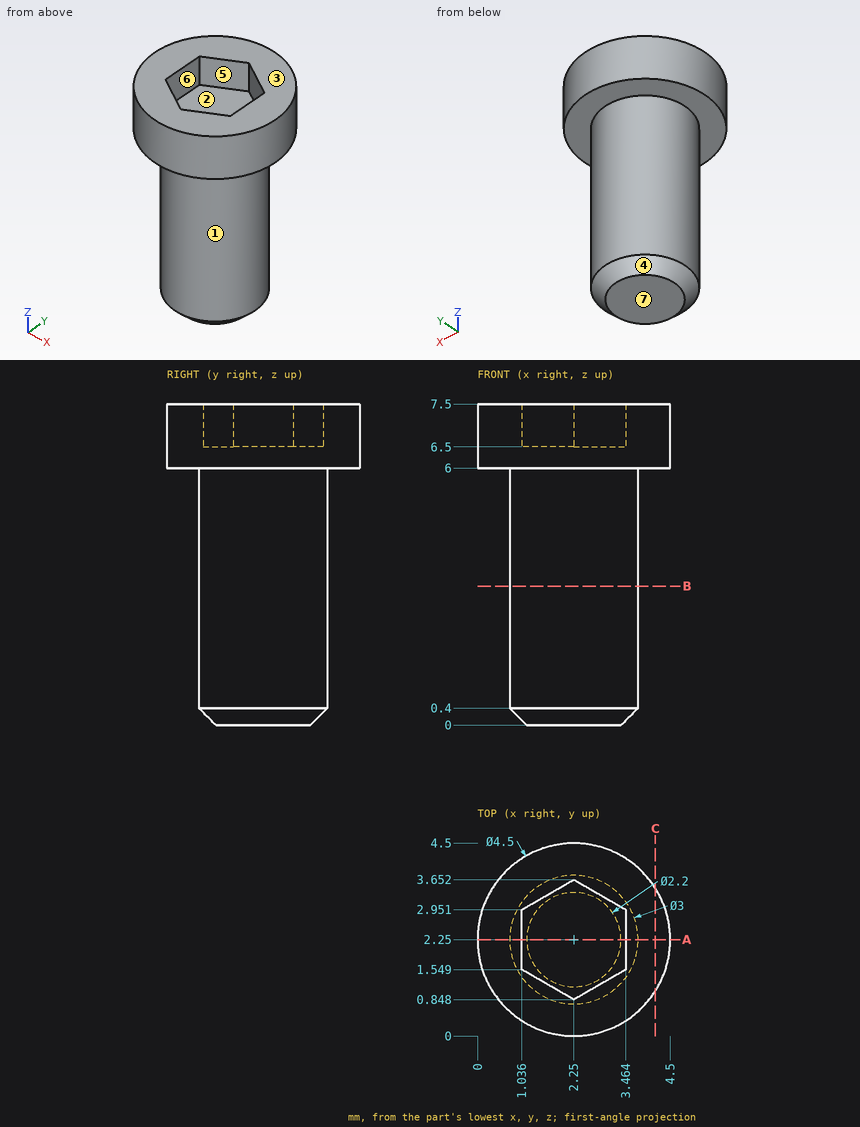
Drawing for the job (mm, zero at the part's lowest x, y, z). A direction names the side the tool comes from. Round coordinates to 2 decimals unless told otherwise and drop trailing zeros. Order: outer loops, then holes, each group sorted by start corner. A loop starts at its lowest first (then second) coordinate and runs counter-clockwise, first axis right, second up. Notation, with made-up numbers: (15.5, -21.75) -> (48.5, -21.75) arc R17 ccw to (48.5, 10.25) -> close; hole circle Ø10 at (75, -28.75). An arc over 180 degrees is marked (long way). Write item = value, one per line. Start each with the question number.
(1) Cut at C-C, the plane x = 4.15. List the corners of the cut face in (y, z) (3 decimals).
(2) Pin check, flat tips, straight feed: P1, Ø1.5, axis at x = 1.5, z = 2.5, coming from the +Y side; P2, Ø1.5, axis at x = 3, z = 4, coming from the -Y side; P3, Ø1, axis at x = 0.5, z = 3.5, coming from the -Y side. Stop position of each tip, or through.
(3) Cut at A-A, the plane y = 2.25. List the corners of the cut face in (x, z), then the cut area to 3 significant figures.
(4) Cut at B-B, the plane z = 3.25. List the corners of the cut face in (x, y), then the cut area to 3 significant figures.
(5) Probe line 1 (Z direction, x = 1.75, y = 3.15); line 2 (Y direction, x = 2.25, z = 5); line 3 (Z direction, x = 3.25, y = 0.45). List the from-to ranges inside material, lowest first. Write a range as [from, to].
(6) Which spindle directions (+Z, -Z, +X, -X, +Y, -Y) get a long thin tool onto all of the face, cutting with end or side? Do the marked faces 1, 2 and 3. Say none if no direction does.
(7) Pull direction X, two halves, no side cores. Call the marked faces 4, 5, 6 and 7: released by +X, released by -X, zero draft, split by the parting line, or undercut.
Model answer:
q1.outline = (1.045, 6) -> (3.455, 6) -> (3.455, 7.5) -> (1.045, 7.5) -> close
q2.P1 = 3.75
q2.P2 = 0.75
q2.P3 = 1.42
q3.outline = (0, 6) -> (0.75, 6) -> (0.75, 0.4) -> (1.15, 0) -> (3.35, 0) -> (3.75, 0.4) -> (3.75, 6) -> (4.5, 6) -> (4.5, 7.5) -> (3.46, 7.5) -> (3.46, 6.5) -> (1.04, 6.5) -> (1.04, 7.5) -> (0, 7.5) -> close
q3.area = 22.2 mm2
q4.outline = circle Ø3 at (2.25, 2.25)
q4.area = 7.07 mm2
q5.line_1 = [0, 6.5]
q5.line_2 = [0.75, 3.75]
q5.line_3 = [6, 7.5]
q6.face_1 = -Z
q6.face_2 = +Z
q6.face_3 = +Z, +X, -X, +Y, -Y
q7.face_4 = split by the parting line
q7.face_5 = undercut
q7.face_6 = undercut
q7.face_7 = zero draft
